Input: dimensioned drawing with shaded views. Units: mm. Origin: part minimum x, y, z. A direction names the side the tool comes from. Give positions to 0.01 mm unless a question says otherwise; leave off trailing zeros. Order: outer loops, then holes, each group sorted by start corner. A loop starts at its lowest first (then second) coordinate and runs counter-clockwise, first axis right, second up. Notation, with made-up numbers: (-22.5, 3) - (4.5, 3) arc R29 ccw to (4.5, 27) - close; hole circle Ø3 at (40, 48). An arc over 180 degrees is marked (long way). Use a Markdown table: item, result.
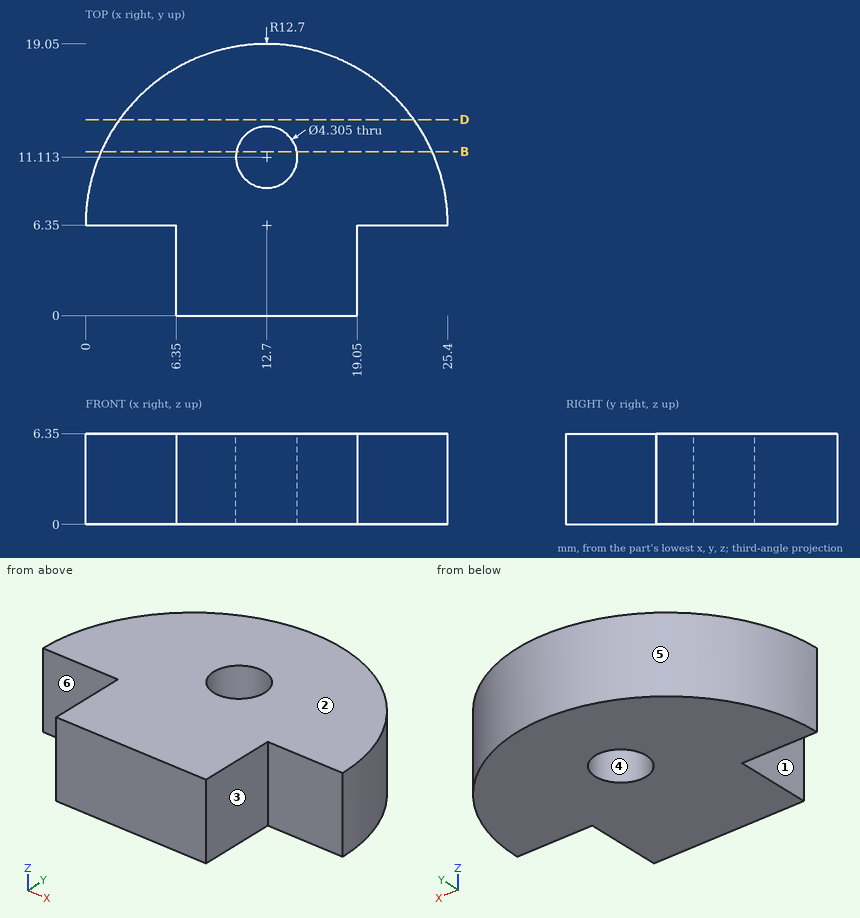
1. Material intervals for line 1 along X through (y, z) = (3.25, 0.75); line 2 along Y through (x, z) = (14, 4.25) (1 decimal); line 3 along X through (y, z) = (11.5, 6), sorted ascending.
Response:
| item | result |
|---|---|
| line 1 | x = 6.35 to 19.05 |
| line 2 | y = 0 to 9.4, 12.8 to 19 |
| line 3 | x = 1.09 to 10.58, 14.82 to 24.31 |
2. Mould query, pull axis Y, two halves, no side actions, for the marked faces 4, 5 and 6. Classes: pulls with the +Y half, pulls with the -Y half, needs draft (parallel to the pull), parting line crosses it, or undercut.
Response:
| item | result |
|---|---|
| face 4 | undercut |
| face 5 | pulls with the +Y half |
| face 6 | pulls with the -Y half |
3. Section query D-D (y = 13.75). Return loops of the section in (x, z).
Response:
| item | result |
|---|---|
| outline | (2.38, 0) - (23.02, 0) - (23.02, 6.35) - (2.38, 6.35) - close |
4. Pin query (flat end, axial travel): pin 1 (1.9 mm diameter, centred on x = 21.5, z = 3, fed in from -Y); pin 2 (3 mm diameter, centred on y = 9, z = 4.5, fed in from +X); pin 3 (2 mm diameter, centred on y = 8, z = 2.5, fed in from +X); pin 4 (2.5 mm diameter, centred on x = 12.7, y = 11.11, fed in from +Z). Return the tip coordinate at first contact, or that it passes through.
Response:
| item | result |
|---|---|
| pin 1 | stops at y = 6.35 |
| pin 2 | stops at x = 25.35 |
| pin 3 | stops at x = 25.38 |
| pin 4 | passes through |
5. Set-up query: the marked faces 1, 2 and 3. Return all of +Z, -Z, +X, -X, +Y, -Y with unobstructed straight access to the full face (end or side cutting, diameter ignored); none if empty.
Response:
| item | result |
|---|---|
| face 1 | +Z, -Z, -X, -Y |
| face 2 | +Z, +X, -X, +Y, -Y |
| face 3 | +Z, -Z, +X, -Y |
6. Section query B-B (y = 11.5). Return loops of the section in (x, z).
Response:
| item | result |
|---|---|
| outline | (1.09, 0) - (10.58, 0) - (10.58, 6.35) - (1.09, 6.35) - close; (14.82, 0) - (24.31, 0) - (24.31, 6.35) - (14.82, 6.35) - close |
